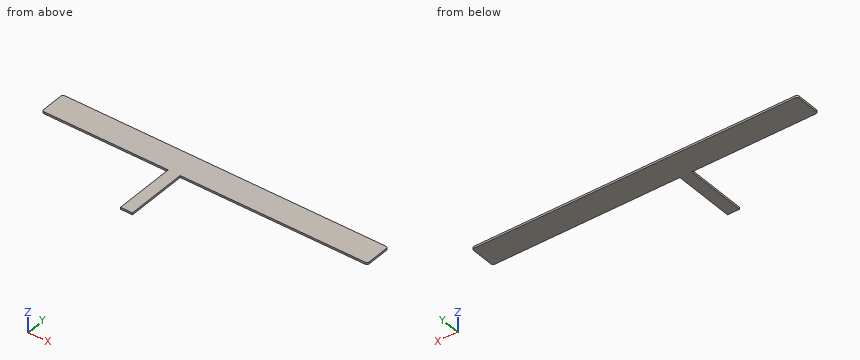
from build123d import *

# Parameters (mm, degrees)
EXTRUDE_1_DEPTH = 0.3
FILLET_1_R      = 0.3


with BuildPart() as part:
    # Sketch 1 → Extrude 1 (new body)
    with BuildSketch(Plane.XY):
        Polygon((-27.107233061, 9.508788635), (21.892766939, 9.508788635), (21.892766939, 5.508788635), (-6.307233061, 5.508788635), (-6.307233061, -3.771211365), (-8.107233061, -3.771211365), (-8.107233061, 5.508788635), (-27.107233061, 5.508788635), align=None)
    extrude(amount=EXTRUDE_1_DEPTH)

    # Fillet 1
    fillet_1_edges = [part.edges().sort_by_distance(p)[0] for p in [
        (21.892766939, 5.508788635, 0.15),
        (21.892766939, 9.508788635, 0.15),
        (-27.107233061, 9.508788635, 0.15),
        (-27.107233061, 5.508788635, 0.15),
    ]]
    fillet(fillet_1_edges, radius=FILLET_1_R)


solid = part.part
Build history of the part. All positions in model axes, mm. Round coordinates to 2 decimals unless told otherwise and drop trailing zeros. Write each loop counter-clockwise with the first axis right and the second up, starting at its lowest first coordinate (ties: lowest second). Pieces come first, ordered by that corner, then holes. Notation, with made-up numbers: M -27,-4.5 L -19,-4.5 A20 ccw -19,26.5 Z; hole C 14,-28.75 d6. An arc over 180 degrees is marked long. Answer in a Markdown table with one row per item.
1. Saw through at B-B (x = -24). List the corners of the cut face in (y, z), and give its area (3 significant figures).
Geometry check:
| item | result |
|---|---|
| outline | M 5.51,0 L 9.51,0 L 9.51,0.3 L 5.51,0.3 Z |
| area | 1.20 mm2 |
2. Saw through at A-A (z = 0.15). List the corners of the cut face in (x, y).
Geometry check:
| item | result |
|---|---|
| outline | M -27.11,5.81 A0.3 ccw -26.81,5.51 L -8.11,5.51 L -8.11,-3.77 L -6.31,-3.77 L -6.31,5.51 L 21.59,5.51 A0.3 ccw 21.89,5.81 L 21.89,9.21 A0.3 ccw 21.59,9.51 L -26.81,9.51 A0.3 ccw -27.11,9.21 Z |
3. Probe L1, parallel to Y at x = 2.5, z = 0.2; L2, parallel to X at y = 0, z = 0.2. List the from-to ranges inside material, lowest first. Write a range as [from, to].
Geometry check:
| item | result |
|---|---|
| L1 | [5.51, 9.51] |
| L2 | [-8.11, -6.31] |
4. Saw through at C-C (y = -0.5). List the corners of the cut face in (x, z).
Geometry check:
| item | result |
|---|---|
| outline | M -8.11,0 L -6.31,0 L -6.31,0.3 L -8.11,0.3 Z |
